Design review of the part built by this model. Coordinates are the model's own, in mm. Coordinates: 2 decimals unless noted, no trailing zeros. Loops run counter-clockwise (first coordinate to the right, second up) from the corner with the lowest first, then second, coordinate; pieces in that order, holes last.
Q1. Wall thickness on probe 1 along Z at (x, y) = (11, 1.1); probe 2 along Z at (x, y) = (-15, 1.05); probe 3 along Z at (x, y) = (46, 1.05): over which ranges is each line inside the solid? List them lowest first.
Q2. Add section D-D on x = 15. Give the boundary of the cut face in (y, z), and give its area (3 significant figures).
Q3. For P1, Ø0.8, axis at x = 24, y = 1, coming from the -Z side; P2, Ø0.7, axis at y = 1, z = -11.5, coming from the -X side; P3, Ø0.7, axis at y = 0.5, z = -11.5, coming from the +X side; P4, Ø4, axis at x = -37.45, z = -11.85, coming from the +Y side, all flat-tipped, find the tip position at first contact; note any pin that passes through.
Q4. Draft analysis for pull direction X (two halves, no side actions). For faces 1 (the face through (25.396, 0.789, -21.614)), 2 (the face through (-41.465, 0.789, -14.571)), 3 (the face through (-35.85, 0.79, -11.92)), state which applies: released by +X, released by -X, zero draft, split by the parting line, or undercut.
Q5. Add section B-B on z = -21.7. Give the boundary of the cut face in (x, y), and give its area (3 significant figures).
Q6. Add section A-A on x = -11. Give the boundary of the cut face in (y, z), and give its area (3 significant figures).
Q7. Add section C-C on y = 1.1. Give the number of separate pieces and of enclosed holes in the cut face, and give its area (3 significant figures).
Autodesk Inventor part; units mm, degrees
ref_plane "YZ Plane" through (0, 0, 0) normal (1, 0, 0) x (0, 1, 0)
ref_plane "XZ Plane" through (0, 0, 0) normal (0, 1, 0) x (-1, 0, 0)
ref_plane "XY Plane" through (0, 0, 0) normal (0, 0, 1) x (1, 0, 0)
sketch "Szkic1" plane through (0, 0, 0) normal (0, 1, 0) x (-1, 0, 0)
  circle A0 centre (-37.45, -11.85) radius 1.6
  circle A1 centre (-11, -21.7) radius 1.55
  circle A2 centre (-15, 31) radius 1.6
  line L0 (-25.3, 6.4859) -> (-22.5, 6.4859)
  line L1 (-22.5, 6.4859) -> (-22.5, -6.4859)
  line L2 (-22.5, -6.4859) -> (-25.3, -6.4859)
  line L3 (-25.3, -6.4859) -> (-25.3, 6.4859)
  line L4 (-42.3, 11.85) -> (-42.3, 11)
  arc A3 (-44.3, 9) -> (-42.3, 11) centre (-44.3, 11) ccw
  line L5 (-44.3, 9) -> (-49.9, 9)
  line L6 (-49.9, 9) -> (-49.9, -9)
  line L7 (-49.9, -9) -> (-44.3, -9)
  arc A4 (-42.3, -11) -> (-44.3, -9) centre (-44.3, -11) ccw
  line L8 (-42.3, -11) -> (-42.3, -11.85)
  arc A5 (-42.3, -11.85) -> (-39.0298, -16.4355) centre (-37.45, -11.85) ccw
  line L9 (-12, -26.7) -> (12, -26.7)
  line L10 (35, 35) -> (-35, 35)
  line L11 (0, -26.7) -> (0, 35)
  line L12 (-49.9, 0) -> (-32, 0)
  circle A6 centre (-37.45, 11.85) radius 1.6
  arc A7 (-42.0609, 13.3541) -> (-42.3, 11.85) centre (-37.45, 11.85) ccw
  line L13 (-35, 35) -> (-42.0609, 13.3541)
  line L14 (-12, -26.7) -> (-39.1714, -16.3842)
  arc A8 (42.3, 11) -> (44.3, 9) centre (44.3, 11) ccw
  line L15 (25.3, 6.4859) -> (22.5, 6.4859)
  line L16 (44.3, 9) -> (49.9, 9)
  line L17 (22.5, 6.4859) -> (22.5, -6.4859)
  line L18 (25.3, -6.4859) -> (25.3, 6.4859)
  line L19 (49.9, 9) -> (49.9, -9)
  line L20 (22.5, -6.4859) -> (25.3, -6.4859)
  line L21 (49.9, -9) -> (44.3, -9)
  arc A9 (44.3, -9) -> (42.3, -11) centre (44.3, -11) ccw
  line L22 (42.3, -11) -> (42.3, -11.85)
  circle A10 centre (37.45, -11.85) radius 1.6
  arc A11 (39.0298, -16.4355) -> (42.3, -11.85) centre (37.45, -11.85) ccw
  circle A12 centre (11, -21.7) radius 1.55
  line L23 (42.3, 11.85) -> (42.3, 11)
  circle A13 centre (15, 31) radius 1.6
  line L24 (49.9, 0) -> (32, 0)
  circle A14 centre (37.45, 11.85) radius 1.6
  arc A15 (42.3, 11.85) -> (42.0609, 13.3541) centre (37.45, 11.85) ccw
  line L25 (35, 35) -> (42.0609, 13.3541)
  line L26 (12, -26.7) -> (39.1714, -16.3842)
  point P0 (0, 0)
  point P1 (-22.5, 0)
  point P2 (-39.0298, 16.4355)
  point P3 (22.5, 0)
  point P4 (39.0298, 16.4355)
  dimension "d5" = 12.9718
  dimension "d6" = 2.8
  dimension "d8" = 22.5
  dimension "d9" = 24
  dimension "d12" = 24.6
  dimension "d13" = 5.6
  dimension "d14" = 5.6
  dimension "d17" = 2.85
  dimension "d18" = 20.2141
  dimension "d19" = 35
extrude "Wyciągnięcie proste1" add sketch "Szkic1" along normal blind 1.6
fillet "Zaokrąglenie1" radius 5 2 edges at (-35, 0.8, 35) (35, 0.8, 35)
fillet "Zaokrąglenie3" radius 1 4 edges at (-49.9, 0.8, -9) (-49.9, 0.8, 9) (49.9, 0.8, 9) (49.9, 0.8, -9)
sketch "Szkic4" plane through (0, 1.6, 0) normal (0, 1, 0) x (1, 0, 0)
  arc A0 (49.9, 8) -> (48.9, 9) centre (48.9, 8) ccw
  line L0 (48.9, 9) -> (44.3, 9)
  arc A1 (42.3, 11) -> (44.3, 9) centre (44.3, 11) ccw
  line L1 (42.3, 11) -> (42.3, 11.85)
  arc A2 (42.3, 11.85) -> (39.1714, 16.3842) centre (37.45, 11.85) ccw
  line L2 (39.1714, 16.3842) -> (12, 26.7)
  line L3 (12, 26.7) -> (-12, 26.7)
  line L4 (-12, 26.7) -> (-39.1714, 16.3842)
  arc A3 (-39.1714, 16.3842) -> (-42.3, 11.85) centre (-37.45, 11.85) ccw
  line L5 (-42.3, 11.85) -> (-42.3, 11)
  arc A4 (-44.3, 9) -> (-42.3, 11) centre (-44.3, 11) ccw
  line L6 (-44.3, 9) -> (-48.9, 9)
  arc A5 (-48.9, 9) -> (-49.9, 8) centre (-48.9, 8) ccw
  line L7 (-49.9, 8) -> (-49.9, -8)
  arc A6 (-49.9, -8) -> (-48.9, -9) centre (-48.9, -8) ccw
  line L8 (-48.9, -9) -> (-44.3, -9)
  arc A7 (-42.3, -11) -> (-44.3, -9) centre (-44.3, -11) ccw
  line L9 (-42.3, -11) -> (-42.3, -11.85)
  arc A8 (-42.3, -11.85) -> (-42.0609, -13.3541) centre (-37.45, -11.85) ccw
  line L10 (-42.0609, -13.3541) -> (-36.1252, -31.5506)
  arc A9 (-36.1252, -31.5506) -> (-31.3717, -35) centre (-31.3717, -30) ccw
  line L11 (-31.3717, -35) -> (31.3717, -35)
  arc A10 (31.3717, -35) -> (36.1252, -31.5506) centre (31.3717, -30) ccw
  line L12 (36.1252, -31.5506) -> (42.0609, -13.3541)
  arc A11 (42.0609, -13.3541) -> (42.3, -11.85) centre (37.45, -11.85) ccw
  line L13 (42.3, -11.85) -> (42.3, -11)
  arc A12 (44.3, -9) -> (42.3, -11) centre (44.3, -11) ccw
  line L14 (44.3, -9) -> (48.9, -9)
  arc A13 (48.9, -9) -> (49.9, -8) centre (48.9, -8) ccw
  line L15 (49.9, -8) -> (49.9, 8)
  line L16 (25.3, -6.4859) -> (22.5, -6.4859)
  line L17 (22.5, -6.4859) -> (22.5, 6.4859)
  line L18 (22.5, 6.4859) -> (25.3, 6.4859)
  line L19 (25.3, 6.4859) -> (25.3, -6.4859)
  circle A14 centre (37.45, 11.85) radius 1.6
  circle A15 centre (11, 21.7) radius 1.55
  circle A16 centre (37.45, -11.85) radius 1.6
  circle A17 centre (15, -31) radius 1.6
  circle A18 centre (-15, -31) radius 1.6
  circle A19 centre (-37.45, 11.85) radius 1.6
  circle A20 centre (-37.45, -11.85) radius 1.6
  circle A21 centre (-11, 21.7) radius 1.55
  line L20 (-25.3, -6.4859) -> (-25.3, 6.4859)
  line L21 (-25.3, 6.4859) -> (-22.5, 6.4859)
  line L22 (-22.5, 6.4859) -> (-22.5, -6.4859)
  line L23 (-22.5, -6.4859) -> (-25.3, -6.4859)
  point P0 (0, 0)
properties part number "plytka_glowna"
Entries:
1. probe 1: z = -26.7 to -23.25, -20.15 to 35
1. probe 2: z = -25.56 to 29.4, 32.6 to 35
1. probe 3: z = -9 to 9
2. outline: (0, -25.56) - (1.6, -25.56) - (1.6, 29.4) - (0, 29.4) - close; (0, 32.6) - (1.6, 32.6) - (1.6, 35) - (0, 35) - close
2. area: 91.8 mm2
3. P1: stops at z = -22.3
3. P2: stops at x = -42.3
3. P3: stops at x = 42.3
3. P4: stops at y = 1.6
4. face 1: released by +X
4. face 2: released by -X
4. face 3: undercut
5. outline: (-25.17, 0) - (-12.55, 0) - (-12.55, 1.6) - (-25.17, 1.6) - close; (-9.45, 0) - (9.45, 0) - (9.45, 1.6) - (-9.45, 1.6) - close; (12.55, 0) - (25.17, 0) - (25.17, 1.6) - (12.55, 1.6) - close
5. area: 70.6 mm2
6. outline: (0, -26.7) - (1.6, -26.7) - (1.6, -23.25) - (0, -23.25) - close; (0, -20.15) - (1.6, -20.15) - (1.6, 35) - (0, 35) - close
6. area: 93.8 mm2
7. separate pieces: 1
7. enclosed holes: 10
7. area: 4,840 mm2
